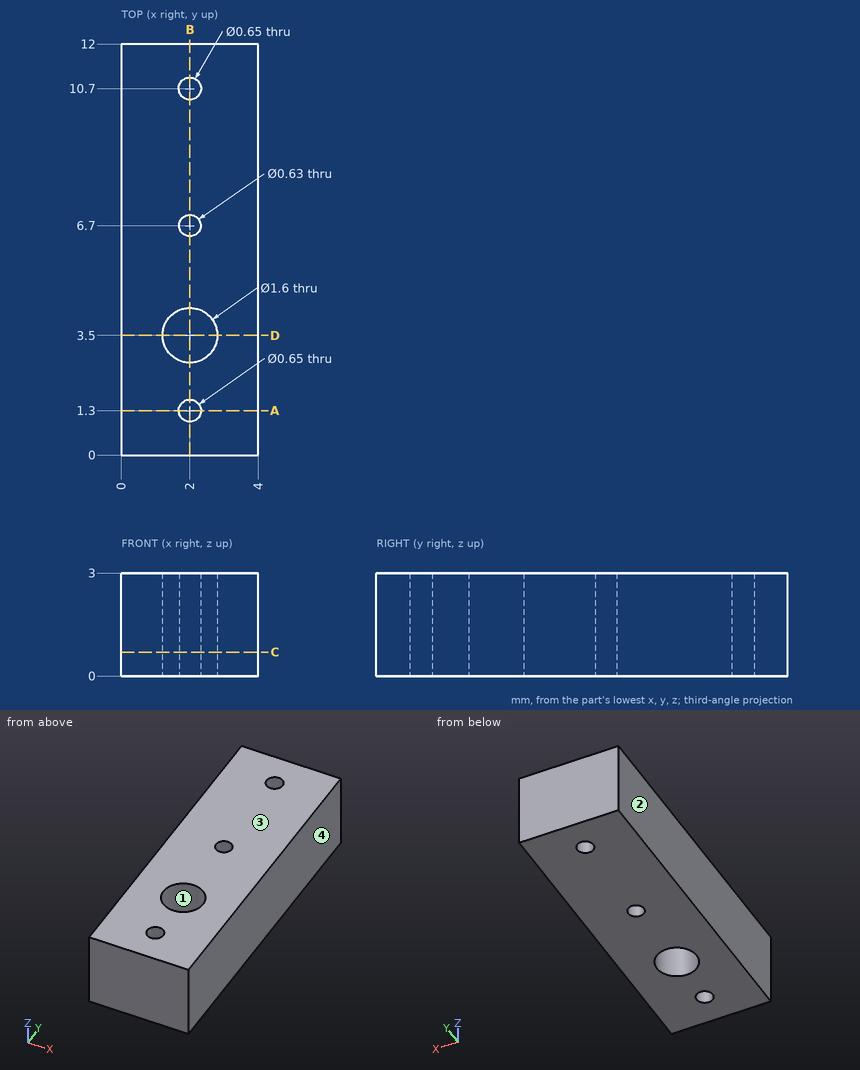
Check sheet for the drawn part. Datum: minimum x, y, z corner. Units: mm. Round coordinates to 2 decimals unless told otherwise and drop trailing zeros. Order: outer loops, then holes, each group sorted by start corner. A loop starts at its lowest first (then second) coordinate and runs counter-clockwise, first axis right, second up.
(1) Scan lines: probe 1 along Y at (x, z) = (2, 1.25) (3 decimals); probe 2 along X at (y, z) = (1.3, 2.35) (3 decimals); probe 3 along X at (y, z) = (4, 1.8). Record each from-to range of solid material in increasing order.
(2) Go/stop test with a flat-tipped pin: P1, Ø1.8, axis at x = 2, y = 3.5, coming from the +Z side. Record where the tip stops, or that it passes through.
(3) Draft check along X on the marked faces 1, 2, 3 and 4. Enter one of: pulls with the +X half, pulls with the -X half, needs draft (parallel to the pull), parting line crosses it, or undercut.
(4) Cross-section at A-A, the plane y = 1.3. Enter the section's corners in (x, z) (3 decimals), and give its area (4 significant figures).
(5) Cross-section at C-C, the plane z = 0.7. Enter the section's corners in (x, y) (3 decimals), and give its area (3 significant figures).
(6) Cross-section at B-B, the plane x = 2. Enter the section's corners in (y, z) (3 decimals).
(7) Cross-section at D-D, the plane y = 3.5. Enter the section's corners in (x, z).
Check sheet entries:
1. probe 1: y = 0 to 0.975, 1.625 to 2.7, 4.3 to 6.385, 7.015 to 10.375, 11.025 to 12
1. probe 2: x = 0 to 1.675, 2.325 to 4
1. probe 3: x = 0 to 1.38, 2.62 to 4
2. P1: stops at z = 3
3. face 1: undercut
3. face 2: pulls with the -X half
3. face 3: needs draft
3. face 4: pulls with the +X half
4. outline: (0, 0) - (1.675, 0) - (1.675, 3) - (0, 3) - close; (2.325, 0) - (4, 0) - (4, 3) - (2.325, 3) - close
4. area: 10.05 mm2
5. outline: (0, 0) - (4, 0) - (4, 12) - (0, 12) - close; hole circle Ø1.6 at (2, 3.5); hole circle Ø0.65 at (2, 1.3); hole circle Ø0.65 at (2, 10.7); hole circle Ø0.63 at (2, 6.7)
5. area: 45.0 mm2
6. outline: (0, 0) - (0.975, 0) - (0.975, 3) - (0, 3) - close; (1.625, 0) - (2.7, 0) - (2.7, 3) - (1.625, 3) - close; (4.3, 0) - (6.385, 0) - (6.385, 3) - (4.3, 3) - close; (7.015, 0) - (10.375, 0) - (10.375, 3) - (7.015, 3) - close; (11.025, 0) - (12, 0) - (12, 3) - (11.025, 3) - close
7. outline: (0, 0) - (1.2, 0) - (1.2, 3) - (0, 3) - close; (2.8, 0) - (4, 0) - (4, 3) - (2.8, 3) - close
